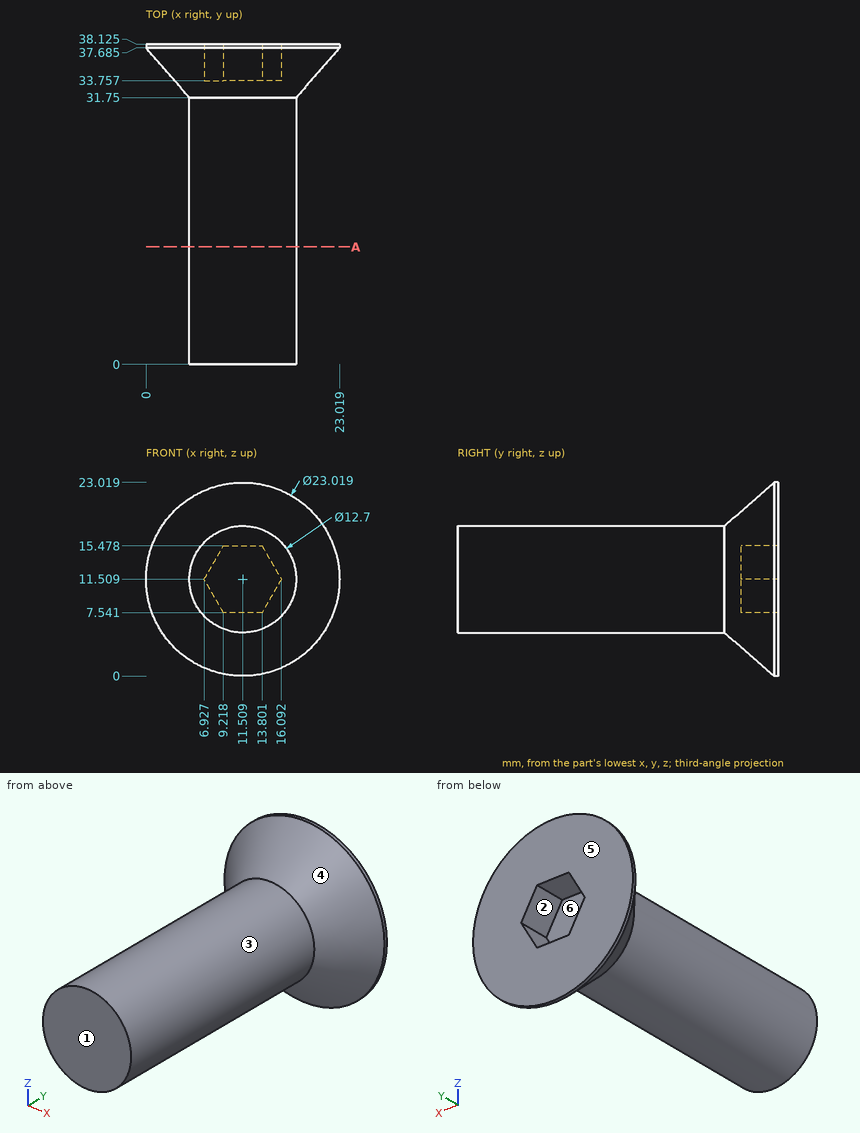
For this review, use the dimensioned drawing (mm, ordinates from the lowest corner) and the shaded views. A direction names the side the tool comes from. Give positions to 0.01 mm unless a question says otherwise; leave off trailing zeros. Order: outer loops, then holes, each group sorted by start corner. A loop starts at its lowest first (then second) coordinate and runs counter-clockwise, first axis right, second up. Notation, with made-up numbers: (-28, 2.5) - (12, 2.5) arc R24 cw to (12, 14.5) - close; hole circle Ø2 at (-30.75, 5). An arc over 180 degrees is marked (long way). Write item = value, one per line. Start each with the question number.
Q1. Mouldability with a two-part tool opening along Z and no side actions: class the marked faces 4, 5 and 6 as released by +Z, released by -Z, zero draft, split by the parting line, or undercut.
Q2. To check wall thickness, follow L1, parallel to X at y = 31, z = 11.25 (1 decimal); L2, parallel to X at y = 34, z = 10 (1 decimal); L3, parallel to Y at x = 11, z = 14.5. State the ranges of each line that lie inside material, in increasing order. Write a range as from..to.
Q3. Tool access review of the marked faces 1, 2 and 3: name each direction out of +Z, -Z, +X, -X, +Y, -Y from which nothing blocks a thin tool from reaching the whole face with its end or side.
Q4. Clearance check with flat-ended pins moving along their axes: pin 1 Ø6 at (y, z) = (22.5, 15) entering from -X; pin 2 Ø1.3 at (x, y) = (11.5, 37) entering from -Z; pin 3 Ø5 at (x, y) = (11, 35) entering from +Z. State where each tip first meets the part, or that it passes through.
Q5. We need section A-A on y = 14. State the section outline as (x, z) points, plus the area to 3 significant figures.
Working result:
q1.face_4 = split by the parting line
q1.face_5 = zero draft
q1.face_6 = undercut
q2.L1 = 5.2..17.9
q2.L2 = 3.3..7.8, 15.2..19.7
q2.L3 = 0..33.76
q3.face_1 = +Z, -Z, +X, -X, -Y
q3.face_2 = +Y
q3.face_3 = -Y
q4.pin_1 = 5.18
q4.pin_2 = 0.03
q4.pin_3 = 22.85
q5.outline = circle Ø12.7 at (11.51, 11.51)
q5.area = 127 mm²
